Source: three-view drawing plus pictorial views. Frame: mm from the lowest corner of the part. Round coordinates to 2 decimals unless told otherwise and drop trailing zeros. Loops run counter-clockwise (first coordinate to the right, second up) from the corner with the lowest first, then second, coordinate; pieces in that order, holes last. Notation, with made-up numbers: M 39,52.25 L 85,52.25 A17 ccw 85,83.25 Z; hole C 33.5,26.5 d3. An arc over 180 degrees is marked long. Return JSON: item names as keys, results as strings. Group by question number.
1) Material intervals for line 1 (X direction, y = 9, z = 9.5); line 2 (X direction, y = 6.5, z = 10.5), sorted ascending. Write a range as from..to.
2) Section C-C (z = 13). Output: boundary loops of the cut face in (x, y), plus the area to 3 significant figures.
3) Section A-A (x = 9). Output: boundary loops of the cut face in (y, z), plus the area to 3 significant figures.
4) Mould query, pull axis Y, two halves, no side actions, for the marked faces 1, 2 and 3. Classes: +Y half, -Y half, draft (parallel to the pull), parting line (faces both ways), or undercut.
5) Contact query for flat-ended pins moving along their axis: P1, Ø4, axis at x = 14.5, z = 10.5, coming from the -Y side; P2, Ø4, axis at x = 13.5, z = 5, coming from the +Y side; P3, Ø5, axis at x = 7.5, z = 11, coming from the -Y side; P4, Ø1, axis at x = 4, z = 2, coming from the -Y side. Output: stop coordinate, or through.
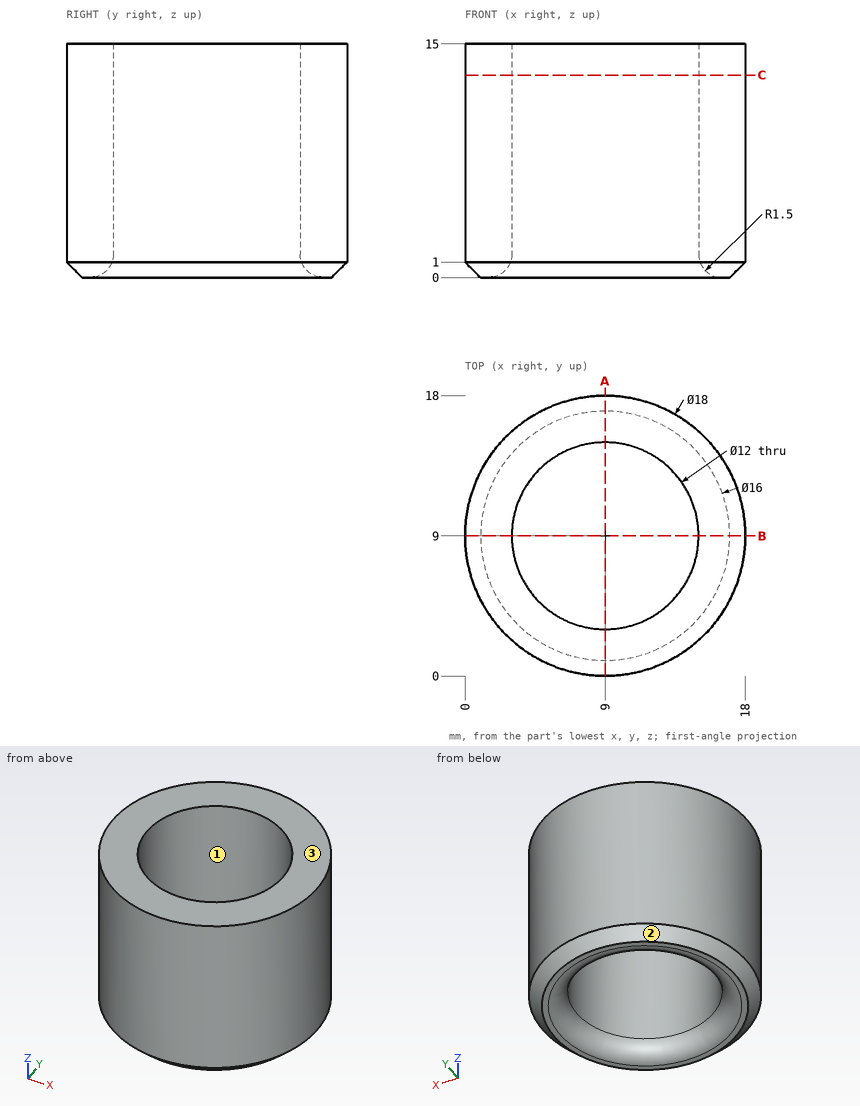
Returned:
{
 "1": {"line 1": "x = 0..3, 15..18", "line 2": "x = 0.35..3.55, 14.45..17.65"},
 "2": {"outline": "C 9,9 d18; hole C 9,9 d12", "area": "141 mm^2"},
 "3": {"outline": "M 0,1 L 1,0 L 1.5,0 A1.5 ccw 3,1.5 L 3,15 L 0,15 Z; M 15,1.5 A1.5 ccw 16.5,0 L 17,0 L 18,1 L 18,15 L 15,15 Z", "area": "88.0 mm^2"},
 "4": {"face 1": "undercut", "face 2": "parting line", "face 3": "draft"},
 "5": {"P1": "stops at y = 0.71", "P2": "stops at y = 17.65", "P3": "stops at y = 0", "P4": "stops at y = 1.21"}
}
